Source: three-view drawing plus pictorial views. Frame: mm from the lowest corner of the part. A direction names the side the tool comes from. Give positions to 0.01 mm unless a question says otherwise; leave off trailing zeros. Order: outer loops, then holes, each group sorted by start corner. A loop starts at its lowest first (then second) coordinate and runs counter-clockwise, first axis right, second up. Notation, with made-up numbers: M 42.25,70 L 81.25,70 A30 ccw 81.25,100 Z; hole C 22.5,81.25 d4. An arc over 180 degrees is marked long. Use CSV: the item, a comma, the result in double quotes. Start each with the question number.
Item 1: First-contact query: pin 1 (1.5 mm diameter, centred on x = 17, y = 13.5, fed in from +Z). Flat tip, straight axial feed; report the tip coordinate or a pass-through.
Item 2: Section query A-A on z = 18.75. Return loops of the section in (x, y), and give its area (3 significant figures).
Item 3: Section query C-C on x = 18.5. Return loops of the section in (y, z), and give its area (4 significant figures).
Item 4: Section query B-B on x = 26.5. Return loops of the section in (y, z), and give its area (3 significant figures).
Item 5: Ray query, probe 1 along Y at (x, z) = (4.5, 13.75); probe 2 along Z at (x, y) = (14, 14.5); probe 3 along Z at (x, y) = (11, 17.75). Return the intervals inside material, ascending. Write a range as from..to.
Item 6: Pull-direction query (Y, two-part tool) for the marked faces 1, 2 and 3; classes: +Y half, -Y half, draft (parallel to the pull), parting line (faces both ways), or undercut.
Item 7: Section query D-D on y = 6.25. Return loops of the section in (x, z), and give its area (3 significant figures).
Item 8: Access query for the marked faces 4, 5 and 6. Directions: +Z, -Z, +X, -X, +Y, -Y. A direction counts if a zero-diameter tool reaches every point of the face in a straight line with its end or side. Return the directions, or none.
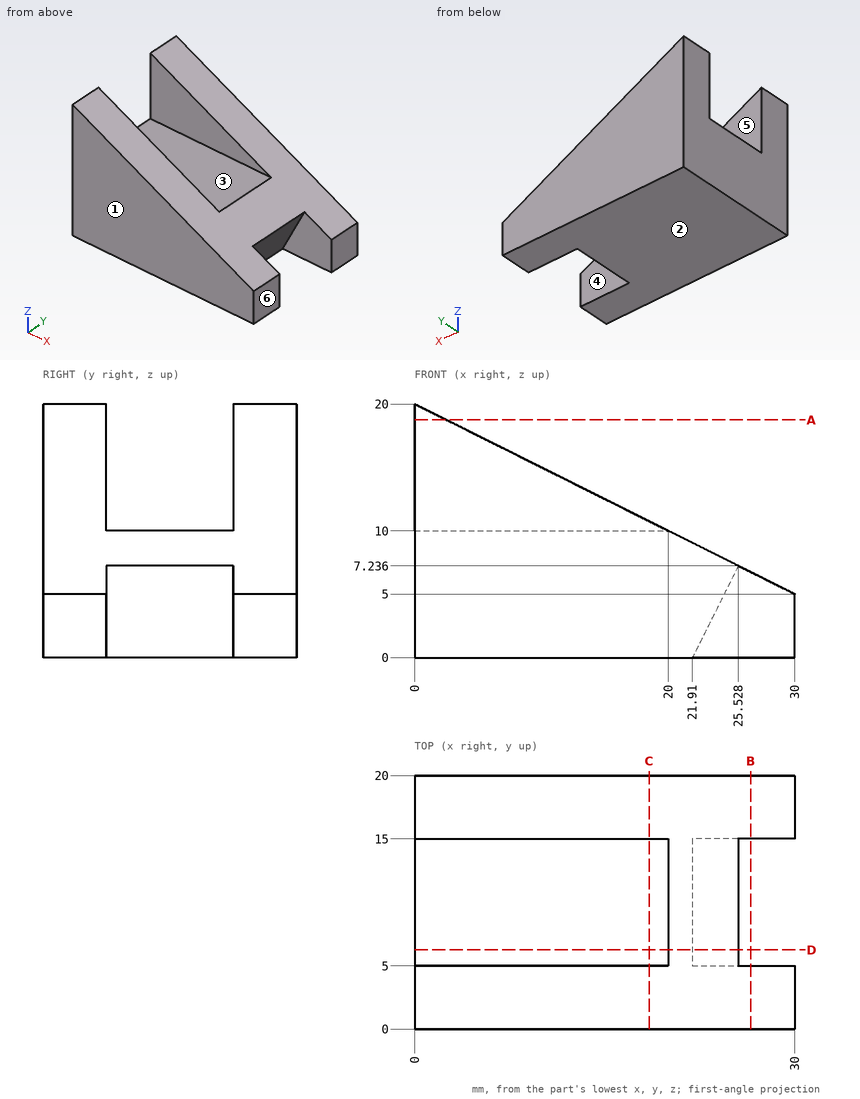
Verdict:
1,pin 1,"z = 10"
2,outline,"M 0,0 L 2.5,0 L 2.5,5 L 0,5 Z; M 0,15 L 2.5,15 L 2.5,20 L 0,20 Z"
2,area,"25.0 mm2"
3,outline,"M 0,0 L 20,0 L 20,10.75 L 15,10.75 L 15,10 L 5,10 L 5,10.75 L 0,10.75 Z"
3,area,"207.5 mm2"
4,outline,"M 0,0 L 5,0 L 5,6.75 L 0,6.75 Z; M 15,0 L 20,0 L 20,6.75 L 15,6.75 Z"
4,area,"67.5 mm2"
5,probe 1,"0..5, 15..20"
5,probe 2,"0..10"
5,probe 3,"0..14.5"
6,face 1,"-Y half"
6,face 2,"draft"
6,face 3,"undercut"
7,outline,"M 0,0 L 21.91,0 L 25.53,7.24 L 20,10 L 0,10 Z"
7,area,"235 mm2"
8,face 4,"-Z, +X"
8,face 5,"+Z, +X, -X"
8,face 6,"+Z, -Z, +X, +Y, -Y"
